Read the model definition and answer for the solid it produces. Units are mm, in the model's axes. Face numbers are marked on the shaded views. A direction names the side the tool comes from. Round coordinates to 2 decimals unless told otherwise and drop trailing zeros. Order: outer loops, then holes, each group sorted by start corner. A loop starts at its lowest first (then second) coordinate and runs counter-clockwise, first axis right, second up. Notation, with made-up numbers: (1.25, 39.5) -> (27.25, 39.5) arc R20 ccw to (27.25, 75.5) -> close; hole circle Ø6 at (37, 51.5). An arc over 180 degrees is marked (long way). One line per item, written item: value. Start each with the question number.
1. Section A-A (y = 28) is taken. Give the vertices of the cut face in (x, z), then the cut area to 3 significant figures.
2. The mould has two halves that part along Z. Classify the marked faces 4, 5, 6 and 7: released by +Z, released by -Z, zero draft, split by the parting line, or undercut.
3. Section C-C (x = -33.5) is taken. Give the vertices of the cut face in (y, z).
4. Flat-ended cylindrical pins translate along their axes: pin 1 Ø12.5 at (x, z) = (-88.9, -166.24) entering from +Y; pin 2 Ø4 at (x, y) = (50.5, 34.5) entering from +Z; pin 3 Ø12.5 at (y, z) = (5.5, -204.5) entering from +X; pin 4 Ø15.5 at (x, z) = (2, -25) entering from +Y. Find the tip coordinate at first contact, or state that the pin passes through.
5. For the marked faces 1, 2 and 3, determine the directions among +Z, -Z, +X, -X, +Y, -Y from which every point of the face is accessible in a straight line to the end or side of a thin tool.
6. Consider line 1 (X direction, y = 4, z = -202); line 2 (X direction, y = 19, z = -171); line 3 (Y direction, x = 72, z = -100). Determine where each line is inside the solid, lowest interval first.
7. Section B-B (z = -60.5) is taken. Give the vertices of the cut face in (x, y), then the cut area to 3 significant figures.
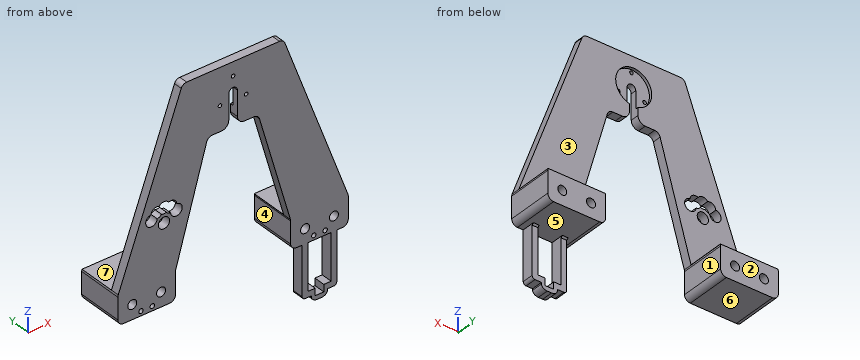
from build123d import *

# Parameters (mm, degrees)
SKETCH1_R            = 3.96875
BOSS_EXTRUDE2_DEPTH  = 40.64
SKETCH4_R            = 1.5875
CUT_EXTRUDE1_DEPTH   = 210.749095026
CUT_EXTRUDE2_START   = 5.08
SKETCH5_R            = 15.875
CUT_EXTRUDE2_DEPTH   = 5.08
SKETCH7_W            = 321.437634852
SKETCH7_H            = 153.081921076
CUT_EXTRUDE3_DEPTH   = 33.02
CUT_EXTRUDE5_DEPTH   = 210.749095026
FILLET1_R            = 6.35
FILLET2_R            = 6.35
EXTRUDE_THIN1_DEPTH  = 10
SKETCH14_R           = 1.950000064
CUT_EXTRUDE6_DEPTH   = 20
BOSS_EXTRUDE4_DEPTH  = 5
MIRROR5_COPY_1_DEPTH = 5
FILLET3_R            = 2.54
SKETCH20_W           = 13.97
SKETCH20_H           = 5.08
BOSS_EXTRUDE5_DEPTH  = 10
FILLET7_SIZE         = 3.81
FILLET7_SIZE_2       = 5.08
FILLET6_SIZE         = 3.81
FILLET6_SIZE_2       = 5.08
CUT_EXTRUDE10_START  = -5
SKETCH19_W           = 7.62
SKETCH19_H           = 10.16
CUT_EXTRUDE10_DEPTH  = 6.27
MIRROR6_OUTLINE_W    = 7.62
MIRROR6_OUTLINE_H    = 5
MIRROR6_DEPTH        = 10
MIRROR6_2_DEPTH      = 10
SKETCH21_W           = 77.087164644
SKETCH21_H           = 69.073945867
CUT_EXTRUDE11_DEPTH  = 210.74909516
SKETCH23_R           = 5.08
CUT_EXTRUDE12_DEPTH  = 255.54404949
SKETCH22_R           = 4.953
CUT_EXTRUDE13_DEPTH  = 255.54404949


# Read off the part's stored shape, not the designer's step: Mirror6
with BuildPart() as part:
    # Sketch1 → Boss-Extrude2 (new body)
    with BuildSketch(Plane(origin=(0, 0, 0), x_dir=(1, 0, 0), z_dir=(0, 1, 0))):
        with BuildLine():
            Line((-96.52, 178.942765331), (-55.88, 178.942765331))
            ThreePointArc((-55.88, 178.942765331), (-52.287897552, 177.454867779), (-50.8, 173.862765331))
            Line((-50.8, 173.862765331), (-50.8, 154.610881096))
            ThreePointArc((-50.8, 154.610881096), (-50.750979429, 153.906859803), (-50.604863787, 153.216425724))
            Line((-50.604863787, 153.216425724), (-23.277092285, 57.485544628))
            ThreePointArc((-23.277092285, 57.485544628), (-21.451849938, 54.824742099), (-18.392228498, 53.8))
            Line((-18.392228498, 53.8), (0, 53.8))
            Line((0, 53.8), (0, 0))
            Line((0, 0), (-40.91748188, 0))
            ThreePointArc((-40.91748188, 0), (-43.817717665, 0.909264766), (-45.679732106, 3.31156205))
            Line((-45.679732106, 3.31156205), (-101.282250226, 153.044327381))
            ThreePointArc((-101.282250226, 153.044327381), (-101.519931557, 153.914386555), (-101.6, 154.812765331))
            Line((-101.6, 154.812765331), (-101.6, 173.862765331))
            ThreePointArc((-101.6, 173.862765331), (-100.112102448, 177.454867779), (-96.52, 178.942765331))
        make_face()
        with Locations(Location((-88.9, 166.242765331, 0), (0, 0, 270))):
            Circle(SKETCH1_R, mode=Mode.SUBTRACT)
        with Locations(Location((-63.5, 166.242765331, 0), (0, 0, 270))):
            Circle(SKETCH1_R, mode=Mode.SUBTRACT)
    boss_extrude2 = extrude(amount=BOSS_EXTRUDE2_DEPTH)

    # Mirror1: Boss-Extrude2 across plane
    add(boss_extrude2.mirror(Plane(origin=(0, 40.64, -53.8), x_dir=(0, 0, 1), z_dir=(-1, 0, 0))))

    # Sketch4 → Cut-Extrude1 (cut, through all)
    with BuildSketch(Plane(origin=(0, 40.64, 0), x_dir=(1, 0, 0), z_dir=(0, 1, 0))):
        with Locations(Location((11.548448759, 32.0195, 0), (0, 0, 270))):
            Circle(SKETCH4_R)
        with Locations(Location((0, 12.017, 0), (0, 0, 270))):
            Circle(SKETCH4_R)
        with Locations(Location((-11.548448759, 32.0195, 0), (0, 0, 270))):
            Circle(SKETCH4_R)
    extrude(amount=-CUT_EXTRUDE1_DEPTH, mode=Mode.SUBTRACT)

    # Sketch5 → Cut-Extrude2 (cut)
    with BuildSketch(Plane(origin=(0, 0, 0), x_dir=(1, 0, 0), z_dir=(0, 1, 0)).offset(CUT_EXTRUDE2_START)):
        with Locations(Location((0, 25.352, 0), (0, 0, 270))):
            Circle(SKETCH5_R)
    extrude(amount=CUT_EXTRUDE2_DEPTH, mode=Mode.SUBTRACT)

    # Sketch7 → Cut-Extrude3 (cut)
    with BuildSketch(Plane(origin=(0, 40.64, 0), x_dir=(1, 0, 0), z_dir=(0, 1, 0))):
        with Locations((5.589227859, 76.540960538)):
            Rectangle(SKETCH7_W, SKETCH7_H)
    extrude(amount=-CUT_EXTRUDE3_DEPTH, mode=Mode.SUBTRACT)

    # Sketch8 → Cut-Extrude5 (cut, through all)
    with BuildSketch(Plane(origin=(0, 0, 0), x_dir=(1, 0, 0), z_dir=(0, 1, 0))):
        with BuildLine():
            Line((-3.81, 25.352), (-3.81, 53.8))
            ThreePointArc((-3.81, 53.8), (0, 57.61), (3.81, 53.8))
            Line((3.81, 53.8), (3.81, 25.352))
            ThreePointArc((3.81, 25.352), (0, 21.542), (-3.81, 25.352))
        make_face()
    extrude(amount=CUT_EXTRUDE5_DEPTH, mode=Mode.SUBTRACT)

    # Fillet1
    fillet1_edges = [part.edges().sort_by_distance(p)[0] for p in [
        (-3.81, 3.81, -53.8),
    ]]
    fillet(fillet1_edges, radius=FILLET1_R)

    # Fillet2
    fillet2_edges = [part.edges().sort_by_distance(p)[0] for p in [
        (3.81, 3.81, -53.8),
    ]]
    fillet(fillet2_edges, radius=FILLET2_R)

    # Sketch9 → Extrude-Thin1 (add)
    with BuildSketch(Plane(origin=(0, 0, 0), x_dir=(1, 0, 0), z_dir=(0, 1, 0))):
        Polygon((-91.44, 173.942765331), (-91.44, 224.742765331), (-60.96, 224.742765331), (-60.96, 173.942765331), (-65.96, 173.942765331), (-65.96, 219.742765331), (-86.44, 219.742765331), (-86.44, 173.942765331), align=None)
    extrude_thin1 = extrude(amount=EXTRUDE_THIN1_DEPTH)

    # Sketch14 → Cut-Extrude6 (cut)
    with BuildSketch(Plane.XZ):
        with Locations(Location((-81.2, -174.942765331, 0), (0, 0, 270))):
            Circle(SKETCH14_R)
        with Locations(Location((-71.2, -174.942765331, 0), (0, 0, 270))):
            Circle(SKETCH14_R)
    cut_extrude6 = extrude(amount=-CUT_EXTRUDE6_DEPTH, mode=Mode.SUBTRACT)

    # Sketch18 → Boss-Extrude4 (add)
    with BuildSketch(Plane(origin=(-60.96, 10, -178.942765331), x_dir=(0, 0, 1), z_dir=(-1, 0, 0))):
        Polygon((-1.27, 0), (0, 1.524), (0, 0), align=None)
    boss_extrude4 = extrude(amount=BOSS_EXTRUDE4_DEPTH)

    # Mirror3: Boss-Extrude4 across plane
    add(boss_extrude4.mirror(Plane(origin=(-76.2, 0, 0), x_dir=(0, 0, 1), z_dir=(1, 0, 0))))

    # Mirror5: Extrude-Thin1, Cut-Extrude6, Boss-Extrude4 across plane
    add(extrude_thin1.mirror(Plane(origin=(0, 0, 0), x_dir=(0, 0, 1), z_dir=(1, 0, 0))))
    add(cut_extrude6.mirror(Plane(origin=(0, 0, 0), x_dir=(0, 0, 1), z_dir=(1, 0, 0))), mode=Mode.SUBTRACT)
    add(boss_extrude4.mirror(Plane(origin=(0, 0, 0), x_dir=(0, 0, 1), z_dir=(1, 0, 0))))

    # Mirror5 copy 1 sketch → Mirror5 copy 1 (add)
    with BuildSketch(Plane(origin=(91.44, 10, -178.942765331), x_dir=(0, 0, 1), z_dir=(-1, 0, 0))):
        Polygon((-1.27, 0), (0, 1.524), (0, 0), align=None)
    extrude(amount=MIRROR5_COPY_1_DEPTH)

    # Fillet3
    fillet3_edges = [part.edges().sort_by_distance(p)[0] for p in [
        (-91.44, 5, -224.742765331),
        (-60.96, 5, -224.742765331),
        (91.44, 5, -224.742765331),
        (60.96, 5, -224.742765331),
    ]]
    fillet(fillet3_edges, radius=FILLET3_R)

    # Sketch20 → Boss-Extrude5 (add)
    with BuildSketch(Plane(origin=(0, 0, 0), x_dir=(1, 0, 0), z_dir=(0, 1, 0))):
        with Locations((-76.2, 227.282765331)):
            Rectangle(SKETCH20_W, SKETCH20_H)
    extrude(amount=BOSS_EXTRUDE5_DEPTH)

    # Fillet7
    # an asymmetric fillet: 5.08, 3.81 mm, written as the material it takes off along each edge
    with BuildSketch(Plane(origin=(-83.185, -12.7, -229.822765331), x_dir=(0, 0, 1), z_dir=(0, 1, 0))) as fillet7_piece_1:
        with BuildLine():
            Bezier((FILLET7_SIZE, 0), (0, 0), (0, FILLET7_SIZE_2), weights=[1, 0.707106781, 1])
            Line((0, FILLET7_SIZE_2), (0, 0))
            Line((0, 0), (FILLET7_SIZE, 0))
        make_face()
    extrude(amount=35.4, mode=Mode.SUBTRACT)

    # Fillet6
    # an asymmetric fillet: 5.08, 3.81 mm, written as the material it takes off along each edge
    with BuildSketch(Plane(origin=(-69.215, -12.7, -229.822765331), x_dir=(0, 0, 1), z_dir=(0, 1, 0))) as fillet6_piece_1:
        with BuildLine():
            Bezier((FILLET6_SIZE, 0), (0, 0), (0, -FILLET6_SIZE_2), weights=[1, 0.707106781, 1])
            Line((0, -FILLET6_SIZE_2), (0, 0))
            Line((0, 0), (FILLET6_SIZE, 0))
        make_face()
    extrude(amount=35.4, mode=Mode.SUBTRACT)

    # Sketch19 → Cut-Extrude10 (cut)
    with BuildSketch(Plane(origin=(0, 0, -224.742765331), x_dir=(-1, 0, 0), z_dir=(0, 0, -1)).offset(CUT_EXTRUDE10_START)):
        with Locations((76.2, 4.92)):
            Rectangle(SKETCH19_W, SKETCH19_H)
    extrude(amount=CUT_EXTRUDE10_DEPTH, mode=Mode.SUBTRACT)

    # Mirror6 outline → Mirror6 (cut)
    with BuildSketch(Plane(origin=(0, 0, 0), x_dir=(1, 0, 0), z_dir=(0, 1, 0))):
        with Locations((76.2, 222.242765331)):
            Rectangle(MIRROR6_OUTLINE_W, MIRROR6_OUTLINE_H)
    extrude(amount=MIRROR6_DEPTH, mode=Mode.SUBTRACT)

    # Mirror6 2 outline → Mirror6 2 (add)
    with BuildSketch(Plane(origin=(0, 0, 0), x_dir=(1, 0, 0), z_dir=(0, 1, 0))):
        with BuildLine():
            add(Edge.make_bspline(
                [(78.105, 229.822765331), (83.185, 229.822765331), (83.185, 226.012765331)],
                knots=[0, 0, 0, 1, 1, 1], degree=2, weights=[1, 0.707106781, 1]))
            Line((78.105, 229.822765331), (74.295, 229.822765331))
            add(Edge.make_bspline(
                [(69.215, 226.012765331), (69.215, 229.822765331), (74.295, 229.822765331)],
                knots=[0, 0, 0, 1, 1, 1], degree=2, weights=[1, 0.707106781, 1]))
            Line((69.215, 226.012765331), (69.215, 224.742765331))
            Line((69.215, 224.742765331), (72.39, 224.742765331))
            Line((72.39, 224.742765331), (72.39, 226.012765331))
            Line((72.39, 226.012765331), (80.01, 226.012765331))
            Line((80.01, 226.012765331), (80.01, 224.742765331))
            Line((80.01, 224.742765331), (83.185, 224.742765331))
            Line((83.185, 224.742765331), (83.185, 226.012765331))
        make_face()
    extrude(amount=MIRROR6_2_DEPTH)

    # Sketch21 → Cut-Extrude11 (cut, through all)
    with BuildSketch(Plane(origin=(0, 0, -178.942765331), x_dir=(-1, 0, 0), z_dir=(0, 0, -1))):
        with Locations((78.752430528, 22.788762469)):
            Rectangle(SKETCH21_W, SKETCH21_H)
    extrude(amount=CUT_EXTRUDE11_DEPTH, mode=Mode.SUBTRACT)

    # Sketch23 → Cut-Extrude12 (cut, through all)
    with BuildSketch(Plane.XZ):
        with Locations((-67.31, -98.573931837)):
            Circle(SKETCH23_R)
        with Locations((-71.958522628, -103.222454465)):
            Circle(SKETCH23_R)
        with Locations((-60.96, -96.872454465)):
            Circle(SKETCH23_R)
        with Locations((-54.61, -98.573931837)):
            Circle(SKETCH23_R)
        with Locations((-49.961477372, -103.222454465)):
            Circle(SKETCH23_R)
    extrude(amount=-CUT_EXTRUDE12_DEPTH, mode=Mode.SUBTRACT)

    # Sketch22 → Cut-Extrude13 (cut, through all)
    with BuildSketch(Plane.XZ):
        with Locations(Location((-60.96, -109.572454465, 0), (0, 0, 270))):
            Circle(SKETCH22_R)
    extrude(amount=-CUT_EXTRUDE13_DEPTH, mode=Mode.SUBTRACT)


solid = part.part
Answer:
1. outline: (-101.6, -173.86) arc R5.08 ccw to (-96.52, -178.94) -> (-55.88, -178.94) arc R5.08 ccw to (-50.8, -173.86) -> (-50.8, -154.61) arc R5.08 cw to (-50.6, -153.22) -> (-50.57, -153.08) -> (-101.3, -153.08) arc R5.08 ccw to (-101.6, -154.81) -> close; (50.57, -153.08) -> (50.6, -153.22) arc R5.08 cw to (50.8, -154.61) -> (50.8, -173.86) arc R5.08 ccw to (55.88, -178.94) -> (96.52, -178.94) arc R5.08 ccw to (101.6, -173.86) -> (101.6, -154.81) arc R5.08 ccw to (101.3, -153.08) -> close; hole circle Ø7.94 at (-88.9, -166.24); hole circle Ø7.94 at (-63.5, -166.24); hole circle Ø7.94 at (63.5, -166.24); hole circle Ø7.94 at (88.9, -166.24)
1. area: 2,410 mm^2
2. face 4: zero draft
2. face 5: undercut
2. face 6: released by -Z
2. face 7: released by +Z
3. outline: (0, -93.3) -> (7.62, -93.3) -> (7.62, 0) -> (0, 0) -> close
4. pin 1: y = 40.64
4. pin 2: z = -153.08
4. pin 3: x = 91.44
4. pin 4: y = 5.08
5. face 1: -Z, +Y, -Y
5. face 2: +Z, -Z, +X, -X, +Y
5. face 3: +Z, +X, -X, +Y
6. line 1: 60.96 to 65.96, 86.44 to 91.44
6. line 2: -101.6 to -50.8, 50.8 to 101.6
6. line 3: 0 to 7.62
7. outline: (-66.92, 0) -> (-24.14, 0) -> (-24.14, 7.62) -> (-66.92, 7.62) -> close; (24.14, 0) -> (66.92, 0) -> (66.92, 7.62) -> (24.14, 7.62) -> close
7. area: 652 mm^2
